Could you check a few things on this drawing? It's one solid part, dimensions in mm from its lowest x, y, z. Coordinates: 2 decimals unless noted, no trailing zeros. Write each loop counter-clockwise with the first axis right and the second up, starting at its lowest first coordinate (ties: lowest second). Pieces come first, ordered by that corner, then holes.
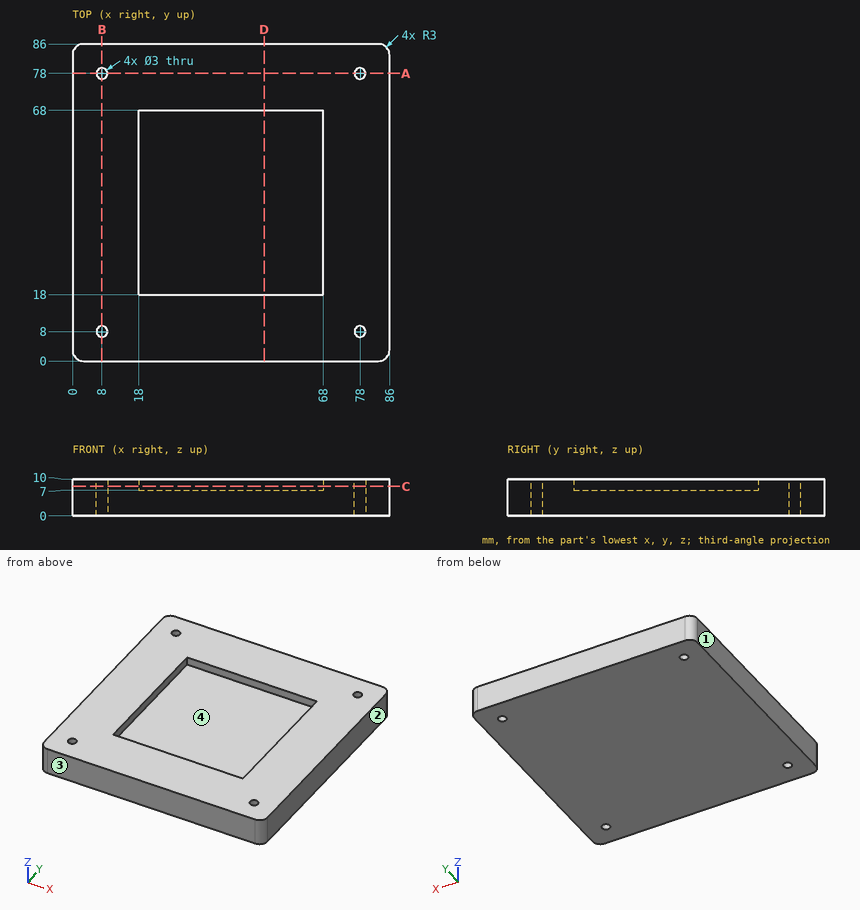
1) Imagine slicing it at C-C on z = 8. Please give me the cut outline in (x, y).
Values follow:
outline: (0, 3) arc R3 ccw to (3, 0) - (83, 0) arc R3 ccw to (86, 3) - (86, 83) arc R3 ccw to (83, 86) - (3, 86) arc R3 ccw to (0, 83) - close; hole circle Ø3 at (8, 8); hole circle Ø3 at (8, 78); hole (18, 18) - (68, 18) - (68, 68) - (18, 68) - close; hole circle Ø3 at (78, 8); hole circle Ø3 at (78, 78)
2) Imagine slicing it at A-A on y = 78. Please give me the cut outline in (x, z).
Values follow:
outline: (0, 0) - (6.5, 0) - (6.5, 10) - (0, 10) - close; (9.5, 0) - (76.5, 0) - (76.5, 10) - (9.5, 10) - close; (79.5, 0) - (86, 0) - (86, 10) - (79.5, 10) - close
3) We'd pull the mould along X, two halves only. Please class the marked faces 1, 2, 3 and 4: pulls with the +X half, pulls with the -X half, needs draft (parallel to the pull), parting line crosses it, or undercut.
Values follow:
face 1: pulls with the -X half
face 2: pulls with the +X half
face 3: needs draft
face 4: undercut
4) Will these pins go through, and if not, where does the flat tip stop? pin 1 (2 mm diameter, centred on x = 54.5, z = 7, fed in from -Y); pin 2 (5 mm diameter, centred on x = 37.5, y = 38, fed in from +Z); pin 3 (2.5 mm diameter, centred on x = 8, y = 8, fed in from +Z).
Values follow:
pin 1: stops at y = 0
pin 2: stops at z = 7
pin 3: passes through
5) Imagine slicing it at D-D on x = 52. Please give me the cut outline in (y, z), then the cut area to 3 significant figures.
Values follow:
outline: (0, 0) - (86, 0) - (86, 10) - (68, 10) - (68, 7) - (18, 7) - (18, 10) - (0, 10) - close
area: 710 mm2
6) I need wall thicknesses on probe 1 along Y at (x, z) = (78, 5.5); probe 2 along Y at (x, z) = (66, 7.75). Which ranges of each line are inside material? Lowest first, please.
Values follow:
probe 1: y = 0 to 6.5, 9.5 to 76.5, 79.5 to 86
probe 2: y = 0 to 18, 68 to 86
